Autodesk Inventor part; units mm, degrees
ref_plane "YZ Plane" through (0, 0, 0) normal (1, 0, 0) x (0, 1, 0)
ref_plane "XZ Plane" through (0, 0, 0) normal (0, 1, 0) x (-1, 0, 0)
ref_plane "XY Plane" through (0, 0, 0) normal (0, 0, 1) x (1, 0, 0)
sketch "Sketch1" plane through (0, 0, 0) normal (0, 0, 1) x (1, 0, 0)
  circle A0 centre (0, 0) radius 5.5
  dimension "d0" = 11
extrude "Extrusion1" add sketch "Sketch1" along normal blind 10
sketch "Sketch2" plane through (0, 0, 10) normal (0, 0, 1) x (1, 0, 0)
  circle A0 centre (0, 0) radius 11.15
  dimension "d3" = 22.3
extrude "Extrusion3" add sketch "Sketch2" along normal blind 44
sketch "Sketch3" plane through (0, 0, 10) normal (0, 0, -1) x (-1, 0, 0)
  circle A0 centre (0, 0) radius 10.15
  circle A1 centre (0, 0) radius 11.15
  dimension "d8" = 20.3
  dimension "d9" = 22.3
extrude "Extrusion4" add sketch "Sketch3" along normal blind 2
sketch "Sketch4" plane through (0, 0, 54) normal (0, 0, 1) x (1, 0, 0)
  circle A0 centre (0, 0) radius 14.15
  dimension "d12" = 28.3
extrude "Extrusion5" add sketch "Sketch4" along normal blind 20
fillet "Fillet1" radius 2 1 edges at (-14.15, 0, 74)
fillet "Fillet2" radius 2 1 edges at (-5.5, 0, 0)
fillet "Fillet3" radius 2 1 edges at (11.15, 0, 8)
fillet "Fillet4" radius 2 1 edges at (-14.15, 0, 54)
properties part number "Elbow_Parallel_Rod_V1"
Verification items for the finished model (mm, model axes). A direction names the side the tool comes from. Coordinates: 2 decimals unless noted, no trailing zeros. Write each loop counter-clockwise with the first axis right and the second up, starting at its lowest first coordinate (ties: lowest second). Pieces come first, ordered by that corner, then holes. Notation, with made-up numbers: M -7.75,1 L 9.25,1 A10 ccw 9.25,5 Z; hole C 61.25,-32.5 d3. An arc over 180 degrees is marked long. Answer as a JSON object with one key per item and string values. Group by question number.
(1) Material ranges on line 1 (Y direction, x = 0, z = 8.5); line 2 (Y direction, x = 0, z = 8.7); line 3 (Z direction, x = 1.5, y = 10), recorded low to high.
(2) Release check for a two-part mould opening along Y. For faces 3 (the face through (-1.19, 5.37, 5.94)), 4 (the face through (0, 0, 0)), 5 (the face through (6.529, 12.553, 63.888)) record: +Y half, -Y half, draft (parallel to the pull), parting line (faces both ways), or undercut.
(3) Cross-section at D-D, the plane z = 59.5. Record the cut outline in (x, y).
(4) Cross-section at C-C, the plane z = 43. Record the cut outline in (x, y).
(5) Cross-section at A-A, the plane y = 0. Record the cut outline in (x, z).
(6) Gauge pin test, flat ends, axial feed: pin 1 (1 mm diameter, centred on x = -2, y = -8.5, fed in from -Z); pin 2 (8 mm diameter, centred on y = 7, z = 16, fed in from -X); pin 3 (4 mm diameter, centred on x = -9, z = 64.5, fed in from -Y). Record the tip position at first contact, or that the pin passes through.
(7) Tool access check on faces 1 (the face through (11, -4, 54)), 2 (the face through (0, 0, 74)). Record the directions out of +Z, -Z, +X, -X, +Y, -Y that give a thin tool (end or side, any length) a straight path to the whole face; none if there is none.
Reply:
{
 "1": {"line 1": "-10.73 to -10.15, -5.5 to 5.5, 10.15 to 10.73", "line 2": "-10.86 to -10.15, -5.5 to 5.5, 10.15 to 10.86", "line 3": "10 to 74"},
 "2": {"face 3": "undercut", "face 4": "draft", "face 5": "parting line"},
 "3": {"outline": "C 0,0 d28.3"},
 "4": {"outline": "C 0,0 d22.3"},
 "5": {"outline": "M -14.15,56 A2 ccw -12.15,54 L -11.15,54 L -11.15,9.73 A2 ccw -10.15,8 L -10.15,10 L -5.5,10 L -5.5,2 A2 ccw -3.5,0 L 3.5,0 A2 ccw 5.5,2 L 5.5,10 L 10.15,10 L 10.15,8 A2 ccw 11.15,9.73 L 11.15,54 L 12.15,54 A2 ccw 14.15,56 L 14.15,72 A2 ccw 12.15,74 L -12.15,74 A2 ccw -14.15,72 Z"},
 "6": {"pin 1": "z = 10", "pin 2": "x = -10.74", "pin 3": "y = -12.3"},
 "7": {"face 1": "-Z", "face 2": "+Z, +X, -X, +Y, -Y"}
}
